Job drawing, mm, ordinate dimensions from the low corner. One solid piece. A direction names the side the tool comes from. Round coordinates to 2 decimals unless told otherwise and drop trailing zeros. Order: outer loops, then holes, each group sorted by start corner. A loop starts at its lowest first (then second) coordinate and runs counter-clockwise, first axis right, second up. Notation, with made-up numbers: (4, 70) - (25, 70) arc R35 ccw to (25, 107) - close; hole circle Ø1 at (81, -7). An arc over 180 degrees is marked (long way). Use one line per item in the form item = value. Start each with the question number.
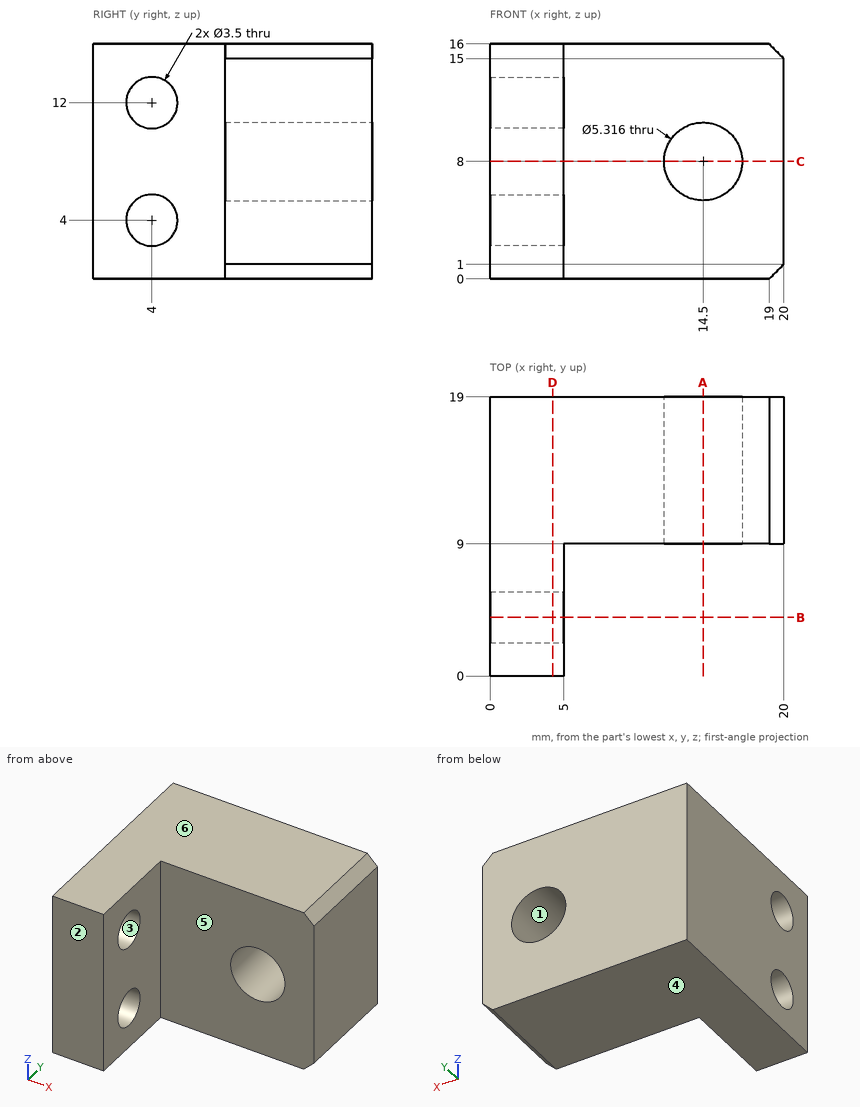
(1) Which spindle directions (+Z, -Z, +X, -X, +Y, -Y) get a long thin tool onto all of the face, cutting with end or side? Do the marked faces 5 and 6. Say none if no direction does.
(2) Flat gauge pins, fed straight in: P1, Ø4, axis at y = 6, z = 11, coming from the +X side; P2, Ø5, axis at x = 14.5, z = 8, coming from the +Y side; P3, Ø8, axis at x = 5, z = 4.5, coming from the -Y side; P4, Ø7.5, axis at x = 14, z = 4.5, coming from the -Y side. Where does each tip first touch, or does it go through?
(3) Mould opens along Z. For the marked faces 1, 2, 3 and 4 say: pulls with the +Z half, pulls with the -Z half, needs draft (parallel to the pull), parting line crosses it, or undercut.
(4) Wall check: line 1 (Z direction, x = 14.5, y = 16.75); line 2 (Y direction, x = 1.85, z = 12); line 3 (X direction, y = 7.5, z = 13). Give the ranges that are in metal, low to high. Write a range as [from, to].
(5) Slice it at C-C (z = 8). Give the cut face in (x, y).
(6) Slice it at A-A (x = 14.5). Give the cut face in (y, z).
(7) Slice it at B-B (y = 4). Give the cut face in (x, z), and give its area (3 significant figures).
(8) Slice it at D-D (x = 4.25). Give the cut face in (y, z), and give its area (3 significant figures).
Results list:
q1.face_5 = +Z, -Z, +X, -Y
q1.face_6 = +Z, +X, -X, +Y, -Y
q2.P1 = 5
q2.P2 = through
q2.P3 = 0
q2.P4 = 9
q3.face_1 = undercut
q3.face_2 = needs draft
q3.face_3 = undercut
q3.face_4 = pulls with the -Z half
q4.line_1 = [0, 5.34], [10.66, 16]
q4.line_2 = [0, 2.25], [5.75, 19]
q4.line_3 = [0, 5]
q5.outline = (0, 0) - (5, 0) - (5, 9) - (11.84, 9) - (11.84, 19) - (0, 19) - close; (17.16, 9) - (20, 9) - (20, 19) - (17.16, 19) - close
q6.outline = (9, 0) - (19, 0) - (19, 5.34) - (9, 5.34) - close; (9, 10.66) - (19, 10.66) - (19, 16) - (9, 16) - close
q7.outline = (0, 0) - (5, 0) - (5, 2.25) - (0, 2.25) - close; (0, 5.75) - (5, 5.75) - (5, 10.25) - (0, 10.25) - close; (0, 13.75) - (5, 13.75) - (5, 16) - (0, 16) - close
q7.area = 45.0 mm²
q8.outline = (0, 0) - (19, 0) - (19, 16) - (0, 16) - close; hole circle Ø3.5 at (4, 4); hole circle Ø3.5 at (4, 12)
q8.area = 285 mm²
